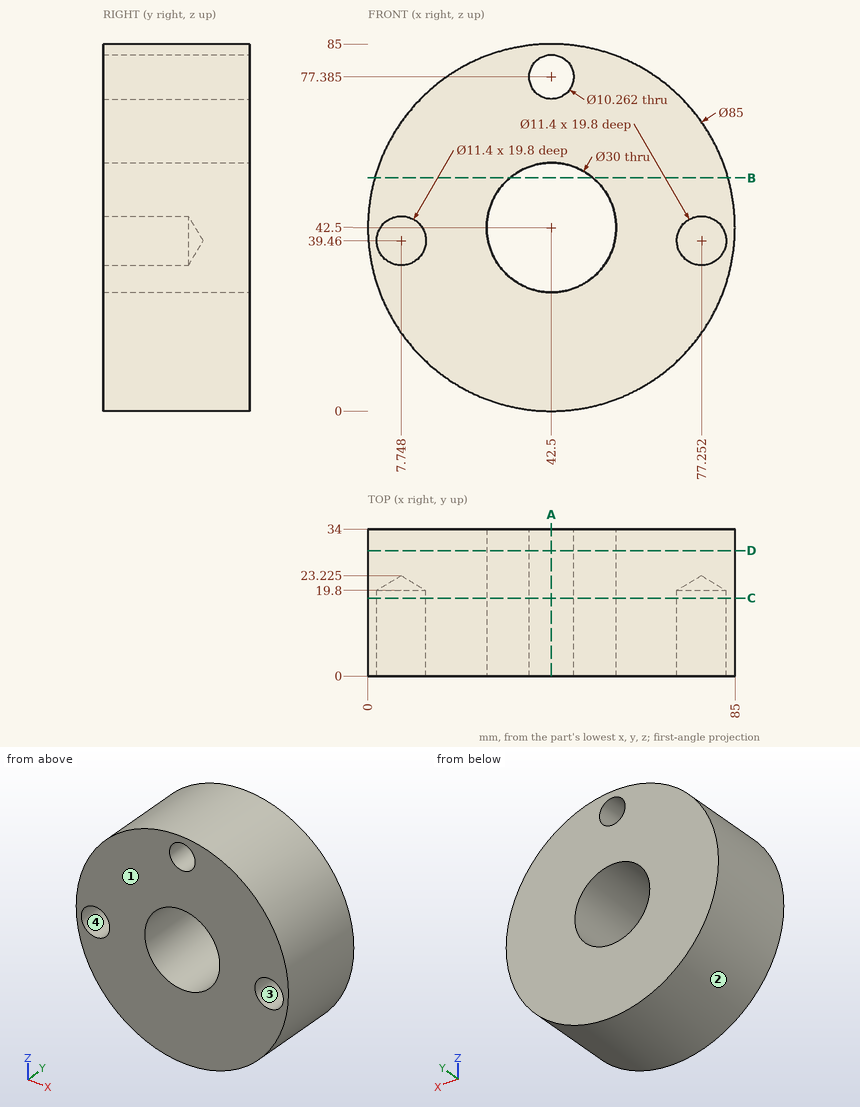
Here's the drawing with two shaded views (mm, measured from the low corner). I have some questions. Coordinates: 2 decimals unless noted, no trailing zeros. Order: outer loops, then holes, each group sorted by start corner. A loop starts at its lowest first (then second) coordinate and runs counter-clockwise, first axis right, second up.
Item 1: If we section it at D-D, the plane y = 29: List the corners of the cut face in (x, z) for me (1 decimal).
Response values:
outline: circle Ø85 at (42.5, 42.5); hole circle Ø30 at (42.5, 42.5); hole circle Ø10.3 at (42.5, 77.4)
Item 2: I'm going to push flat-ended pins straight in: pin 1 Ø18 at (x, z) = (42.5, 42.5) entering from +Y; pin 2 Ø8 at (y, z) = (13.5, 22.5) entering from -X; pin 3 Ø4 at (x, y) = (69.5, 20) entering from -Z; pin 4 Ø3 at (y, z) = (6.5, 71) entering from +X. Where does each tip first touch, or does it pass through?
Response values:
pin 1: passes through
pin 2: stops at x = 3.13
pin 3: stops at z = 8.13
pin 4: stops at x = 75.32
Item 3: Thinking about a two-plate mould opening in X: for the marked faces 1, 2, 3 and 4, which applies, pulls with the +X half, pulls with the -X half, needs draft (parallel to the pull), parting line crosses it, or undercut?
Response values:
face 1: needs draft
face 2: parting line crosses it
face 3: undercut
face 4: undercut
Item 4: If we section it at A-A, the plane x = 42.5: List the corners of the cut face in (y, z) for me.
Response values:
outline: (0, 0) - (34, 0) - (34, 27.5) - (0, 27.5) - close; (0, 57.5) - (34, 57.5) - (34, 72.25) - (0, 72.25) - close; (0, 82.52) - (34, 82.52) - (34, 85) - (0, 85) - close
Item 5: If we section it at B-B, the plane z = 54: List the corners of the cut face in (x, y) for me (1 decimal).
Response values:
outline: (1.6, 0) - (32.9, 0) - (32.9, 34) - (1.6, 34) - close; (52.1, 0) - (83.4, 0) - (83.4, 34) - (52.1, 34) - close
Item 6: I need wall thicknesses on probe 1 along Z at (x, y) = (42, 25); probe 2 along Z at (x, y) = (41.5, 18.5); probe 3 along X at (y, z) = (26, 42). Which ranges of each line are inside material? Lowest first, please.
Response values:
probe 1: z = 0 to 27.51, 57.49 to 72.28, 82.49 to 85
probe 2: z = 0.01 to 27.53, 57.47 to 72.35, 82.42 to 84.99
probe 3: x = 0 to 27.51, 57.49 to 85
Item 7: If we section it at C-C, the plane y = 18: List the corners of the cut face in (x, z) for me (1 decimal).
Response values:
outline: circle Ø85 at (42.5, 42.5); hole circle Ø11.4 at (7.7, 39.5); hole circle Ø30 at (42.5, 42.5); hole circle Ø10.3 at (42.5, 77.4); hole circle Ø11.4 at (77.3, 39.5)
